from build123d import *

# Parameters (mm, degrees)
SKETCH2_R          = 1.5
CUT_EXTRUDE1_DEPTH = 6.338539126


with BuildPart() as part:
    # Sketch1 → Revolve1 (revolve)
    with BuildSketch(Plane.XY):
        Polygon((0, 2), (0, 0), (-2, 0), (-2, 1), (-2.5, 1), (-2.5, 2), align=None)
    revolve1 = revolve(axis=Axis((0, 2, 0), (0, -1, 0)))

    # Mirror1: Revolve1 across plane
    add(revolve1.mirror(Plane(origin=(-2, 0, 0), x_dir=(0, 0, 1), z_dir=(0, -1, 0))))

    # Sketch2 → Cut-Extrude1 (cut, through all)
    with BuildSketch(Plane(origin=(0, 2, 0), x_dir=(1, 0, 0), z_dir=(0, 1, 0))):
        with Locations(Location((0, 0, 0), (0, 0, 180))):
            Circle(SKETCH2_R)
    extrude(amount=-CUT_EXTRUDE1_DEPTH, mode=Mode.SUBTRACT)


solid = part.part
Read the model definition and answer for the solid it produces. Units are mm, in the model's axes. A direction names the side the tool comes from. Round coordinates to 2 decimals unless told otherwise and drop trailing zeros. Write each loop counter-clockwise with the first axis right and the second up, starting at its lowest first coordinate (ties: lowest second). Pieces come first, ordered by that corner, then holes. Notation, with made-up numbers: (-8, 13) - (23, 13) arc R24 cw to (23, 24) - close; hole circle Ø10 at (74.25, -9.75). An arc over 180 degrees is marked (long way). Use a Markdown table: item, result.
(1) The part is cut by section C-C (y = -1.2). Write down the section's boundary in (x, z).
Reported:
| item | result |
|---|---|
| outline | circle Ø5 at (0, 0); hole circle Ø3 at (0, 0) |
(2) The part is cut by section B-B (x = 0). Write down the section's boundary in (y, z).
Reported:
| item | result |
|---|---|
| outline | (-2, -2.5) - (-1, -2.5) - (-1, -2) - (1, -2) - (1, -2.5) - (2, -2.5) - (2, -1.5) - (-2, -1.5) - close; (-2, 1.5) - (2, 1.5) - (2, 2.5) - (1, 2.5) - (1, 2) - (-1, 2) - (-1, 2.5) - (-2, 2.5) - close |
(3) The part is cut by section A-A (z = 0). Write down the section's boundary in (x, y).
Reported:
| item | result |
|---|---|
| outline | (-2.5, -2) - (-1.5, -2) - (-1.5, 2) - (-2.5, 2) - (-2.5, 1) - (-2, 1) - (-2, -1) - (-2.5, -1) - close; (1.5, -2) - (2.5, -2) - (2.5, -1) - (2, -1) - (2, 1) - (2.5, 1) - (2.5, 2) - (1.5, 2) - close |
(4) Straight lines are drawn through the part: line 1 along Y through (x, z) = (-1.05, 1.75); line 2 along Z through (x, y) = (0, 1.15); line 3 along Z through (x, y) = (0, 0.8). For each, find the intervals that lie inside material, in ascending order. Write a range as [from, to].
Reported:
| item | result |
|---|---|
| line 1 | [-2, -1], [1, 2] |
| line 2 | [-2.5, -1.5], [1.5, 2.5] |
| line 3 | [-2, -1.5], [1.5, 2] |
(5) Which of the six approach directions +Z, -Z, +X, -X, +Y, -Y give full straight-line access (tool end or side, diameter ignored) to faces 4 (the flat face through (-1, -1, -2)), 5 (the cylindrical face through (0.54, 1.51, 2.44))?
Reported:
| item | result |
|---|---|
| face 4 | none |
| face 5 | +Y, -Y |
(6) The mould has two halves that part along Y. Classify faces 1 (the flat face through (-2, 2, 0)), 2 (the flat face through (-1, 1, -2)), 3 (the flat face through (-2, -2, 0)): released by +Y, released by -Y, zero draft, split by the parting line, or undercut.
Reported:
| item | result |
|---|---|
| face 1 | released by +Y |
| face 2 | undercut |
| face 3 | released by -Y |
(7) Each of these flat-tipped pins is pushed along its axis until it touches: pin 1 Ø1 at (y, z) = (0, 0) entering from -X; pin 2 Ø1.5 at (y, z) = (-0.5, -2) entering from +X. Where does it stop, or does it pass through?
Reported:
| item | result |
|---|---|
| pin 1 | x = -2 |
| pin 2 | x = 2.04 |
